Could you check a few things on this model? Use its own coordinates, in mm. A direction names the side the tool comes from. Give positions to 0.01 mm unless a question says otherwise; leave off trailing zeros. Order: outer loops, then holes, each group sorted by start corner. A loop starts at its lowest first (then second) coordinate and runs counter-clockwise, first axis right, second up.
from build123d import *

# Parameters (mm, degrees)
BOSS_EXTRUDE1_DEPTH = 45
SKETCH2_W           = 5
SKETCH2_H           = 20
BOSS_EXTRUDE3_DEPTH = 40
SKETCH3_R           = 1.925
CUT_EXTRUDE1_DEPTH  = 200
SKETCH4_R           = 11.15
CUT_EXTRUDE2_DEPTH  = 200
SKETCH5_R           = 1.4
CUT_EXTRUDE3_DEPTH  = 200
FILLET1_R           = 2


with BuildPart() as part:
    # Sketch1 → Boss-Extrude1 (new body)
    with BuildSketch(Plane.XY):
        Polygon((26.25, 0), (-26.25, 0), (-26.25, 20), (-21.25, 20), (-21.25, 5), (21.25, 5), (21.25, 20), (26.25, 20), align=None)
    extrude(amount=BOSS_EXTRUDE1_DEPTH)

    # Sketch2 → Boss-Extrude3 (add, symmetric)
    with BuildSketch(Plane(origin=(0, 0, 0), x_dir=(0, 0, -1), z_dir=(1, 0, 0))):
        with Locations((2.5, 10)):
            Rectangle(SKETCH2_W, SKETCH2_H)
    extrude(amount=BOSS_EXTRUDE3_DEPTH, both=True)

    # Sketch3 → Cut-Extrude1 (cut)
    with BuildSketch(Plane.XY):
        with Locations((-33.125, 10)):
            Circle(SKETCH3_R)
        with Locations(Location((33.125, 10, 0), (0, 0, 270))):
            Circle(SKETCH3_R)
    extrude(amount=-CUT_EXTRUDE1_DEPTH, mode=Mode.SUBTRACT)

    # Sketch4 → Cut-Extrude2 (cut)
    with BuildSketch(Plane(origin=(0, 5, 0), x_dir=(1, 0, 0), z_dir=(0, 1, 0))):
        with Locations(Location((0, -22.5, 0), (0, 0, 270))):
            Circle(SKETCH4_R)
    extrude(amount=-CUT_EXTRUDE2_DEPTH, mode=Mode.SUBTRACT)

    # Sketch5 → Cut-Extrude3 (cut)
    with BuildSketch(Plane(origin=(0, 5, 0), x_dir=(1, 0, 0), z_dir=(0, 1, 0))):
        with Locations(Location((-15.5, -7, 0), (0, 0, 270))):
            Circle(SKETCH5_R)
        with Locations(Location((15.5, -7, 0), (0, 0, 270))):
            Circle(SKETCH5_R)
        with Locations(Location((-15.5, -38, 0), (0, 0, 270))):
            Circle(SKETCH5_R)
        with Locations(Location((15.5, -38, 0), (0, 0, 270))):
            Circle(SKETCH5_R)
    extrude(amount=-CUT_EXTRUDE3_DEPTH, mode=Mode.SUBTRACT)

    # Fillet1
    fillet1_edges = [part.edges().sort_by_distance(p)[0] for p in [
        (-26.25, 10, 0),
        (26.25, 10, 0),
    ]]
    fillet(fillet1_edges, radius=FILLET1_R)


solid = part.part
Item 1: Imagine slicing it at D-D on x = -15.5. List the corners of the cut face in (y, z) for me.
Findings:
outline: (0, -5) - (20, -5) - (20, 0) - (5, 0) - (5, 5.6) - (0, 5.6) - close; (0, 8.4) - (5, 8.4) - (5, 36.6) - (0, 36.6) - close; (0, 39.4) - (5, 39.4) - (5, 45) - (0, 45) - close
Item 2: Imagine slicing it at C-C on y = 11. List the corners of the cut face in (x, z) for me, then the cut area to 3 significant figures.
Findings:
outline: (-40, -5) - (-34.77, -5) - (-34.77, 0) - (-40, 0) - close; (-31.48, -5) - (31.48, -5) - (31.48, 0) - (28.25, 0) arc R2 cw to (26.25, 2) - (26.25, 45) - (21.25, 45) - (21.25, 0) - (-21.25, 0) - (-21.25, 45) - (-26.25, 45) - (-26.25, 2) arc R2 cw to (-28.25, 0) - (-31.48, 0) - close; (34.77, -5) - (40, -5) - (40, 0) - (34.77, 0) - close
area: 819 mm2
Item 3: Please list where these lines run through material, in increasing order: line 1 along X through (y, z) = (3.4, 38); line 2 along X through (y, z) = (5.75, 3.5); line 3 along Z through (x, y) = (-20.5, 18.5).
Findings:
line 1: x = -26.25 to -16.9, -14.1 to 14.1, 16.9 to 26.25
line 2: x = -26.25 to -21.25, 21.25 to 26.25
line 3: z = -5 to 0
Item 4: For pin 1 (13 mm diameter, centred on x = -5, z = 16.5, fed in from +Y); pin 2 (6 mm diameter, centred on y = 14, z = 14, fed in from +X); pin 3 (12 mm diameter, centred on x = 15, y = 12.5, fed in from +Z), each with a flat end and sliding along its axis, tell me the tip position at first contact or that it passes through.
Findings:
pin 1: stops at y = 5
pin 2: stops at x = 26.25
pin 3: stops at z = 0
Item 5: For faces 5 (the flat face through (-5, 5, 12)), 6 (the flat face through (-26.25, 10, 23)), 7 (the flat face through (26.25, 10, 23)), which set-ups out of +Z, -Z, +X, -X, +Y, -Y let a thin tool reach every point of the face, with its end or its side?
Findings:
face 5: +Z, +Y
face 6: +Z, -X, +Y, -Y
face 7: +Z, +X, +Y, -Y
Item 6: Imagine slicing it at A-A on z = 22.5. List the corners of the cut face in (x, y) for me.
Findings:
outline: (-26.25, 0) - (-11.15, 0) - (-11.15, 5) - (-21.25, 5) - (-21.25, 20) - (-26.25, 20) - close; (11.15, 0) - (26.25, 0) - (26.25, 20) - (21.25, 20) - (21.25, 5) - (11.15, 5) - close
Item 7: Imagine slicing it at B-B on x = 0. List the corners of the cut face in (y, z) for me.
Findings:
outline: (0, -5) - (20, -5) - (20, 0) - (5, 0) - (5, 11.35) - (0, 11.35) - close; (0, 33.65) - (5, 33.65) - (5, 45) - (0, 45) - close
Item 8: We'd pull the mould along Y, two halves only. Please class faces 1 (the flat face through (0.2, 20, -0.3)), 2 (the flat face through (-8.3, 0, 14.8)), 3 (the flat face through (40, 10, -2)), 4 (the cylindrical face through (-31.35, 9.26, -2.46)): +Y half, -Y half, draft (parallel to the pull), parting line (faces both ways), or undercut.
Findings:
face 1: +Y half
face 2: -Y half
face 3: draft
face 4: undercut
